The listing builds one solid part. Answer for the finished solid, in the listing's coordinates (mm). Give positions to 0.01 mm unless a question says otherwise; leave off trailing zeros. Order: outer loops, then holes, each group sorted by start corner. A loop starts at its lowest first (then second) coordinate and runs counter-clockwise, first axis right, second up. Notation, with made-up numbers: (10.5, 58.5) - (25.5, 58.5) arc R5 ccw to (25.5, 64.5) - close; hole circle Ø2 at (52.25, 78.5). An arc over 180 degrees is marked (long way). Use a Markdown table: item, result. Add a question column.
1) Flat-ended cylindrical pins translate along their axes: pin 1 (0.9 mm diameter, centred on y = 1.5, z = 76, fed in from -X); pin 2 (1.5 mm diameter, centred on x = 59, y = 1.5, fed in from +Z). Find the tip coordinate at first contact, or state that the pin passes through.
2) Find section B-B, the plane x = -76. Determine the outline of the cut face in (y, z).
3) Find section D-D, the plane x = 128. Determine the outline of the cut face in (y, z), plus the area to 3 significant figures.
4) Straight lines are drawn through the part: line 1 (Z direction, x = -19, y = 2.55); line 2 (X direction, y = 1.05, z = -57); line 3 (Z direction, x = 48.5, y = 0.5). For each, find the intervals that lie inside material, in ascending order.
5) Find section C-C, the plane x = 47.5. Determine the outline of the cut face in (y, z), plus the area to 3 significant figures.
6) Find section A-A, the plane y = 0.45. Determine the outline of the cut face in (x, z), plus the area to 3 significant figures.
from build123d import *

# Parameters (mm, degrees)
SKETCH_1_R      = 165
EXTRUDE_1_DEPTH = 3


with BuildPart() as part:
    # 草图1 → 凸台-拉伸1 (new body)
    with BuildSketch(Plane(origin=(0, 0, 0), x_dir=(1, 0, 0), z_dir=(0, 1, 0))):
        with Locations(Location((0, 0, 0), (0, 0, 270))):
            Circle(SKETCH_1_R)
        with BuildLine():
            Line((-15, 98.868599666), (-15, 15))
            Line((-15, 15), (-98.868599666, 15))
            ThreePointArc((-98.868599666, 15), (-70.710678119, 70.710678119), (-15, 98.868599666))
        make_face(mode=Mode.SUBTRACT)
        with BuildLine():
            Line((15, 98.868599666), (15, 15))
            Line((15, 15), (98.868599666, 15))
            ThreePointArc((98.868599666, 15), (70.710678119, 70.710678119), (15, 98.868599666))
        make_face(mode=Mode.SUBTRACT)
        with BuildLine():
            Line((-98.868599666, -15), (-15, -15))
            Line((-15, -15), (-15, -98.868599666))
            ThreePointArc((-15, -98.868599666), (-70.710678119, -70.710678119), (-98.868599666, -15))
        make_face(mode=Mode.SUBTRACT)
        with BuildLine():
            Line((15, -15), (15, -98.868599666))
            ThreePointArc((15, -98.868599666), (70.710678119, -70.710678119), (98.868599666, -15))
            Line((98.868599666, -15), (15, -15))
        make_face(mode=Mode.SUBTRACT)
    extrude(amount=EXTRUDE_1_DEPTH)


solid = part.part
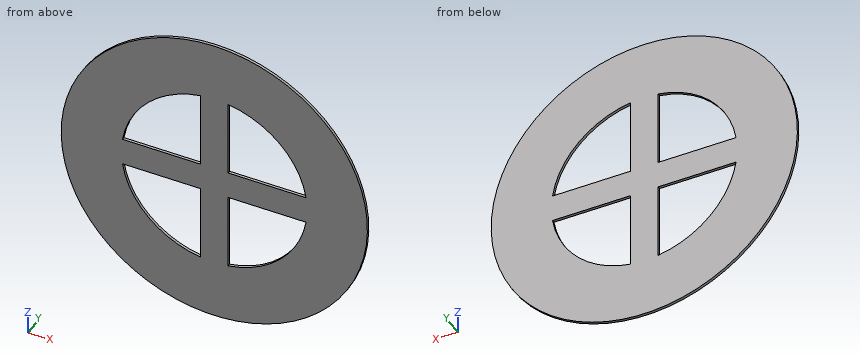
The answers:
| question | item | result |
|---|---|---|
| 1 | pin 1 | x = -146.69 |
| 1 | pin 2 | z = 154.38 |
| 2 | outline | (0, -146.45) - (3, -146.45) - (3, -64.99) - (0, -64.99) - close; (0, -15) - (3, -15) - (3, 15) - (0, 15) - close; (0, 64.99) - (3, 64.99) - (3, 146.45) - (0, 146.45) - close |
| 3 | outline | (0, -104.12) - (3, -104.12) - (3, 104.12) - (0, 104.12) - close |
| 3 | area | 625 mm2 |
| 4 | line 1 | -163.9 to -98.18, -15 to 15, 98.18 to 163.9 |
| 4 | line 2 | -154.84 to -82.16, -15 to 15, 82.16 to 154.84 |
| 4 | line 3 | -157.71 to -87.45, -15 to 15, 87.45 to 157.71 |
| 5 | outline | (0, -158.02) - (3, -158.02) - (3, -88) - (0, -88) - close; (0, -15) - (3, -15) - (3, 15) - (0, 15) - close; (0, 88) - (3, 88) - (3, 158.02) - (0, 158.02) - close |
| 5 | area | 510 mm2 |
| 6 | outline | circle Ø330 at (0, 0); hole (-98.87, -15) arc R100 ccw to (-15, -98.87) - (-15, -15) - close; hole (-98.87, 15) - (-15, 15) - (-15, 98.87) arc R100 ccw to start; hole (15, -98.87) arc R100 ccw to (98.87, -15) - (15, -15) - close; hole (15, 15) - (98.87, 15) arc R100 ccw to (15, 98.87) - close |
| 6 | area | 65,200 mm2 |
